```python
from build123d import *

# Parameters (mm, degrees)
BOSS_EXTRUDE1_DEPTH     = 3
BOSS_EXTRUDE1_2_DEPTH   = 3
BOSS_EXTRUDE2_START     = 1.2
SKETCH3_R               = 16.55
SKETCH3_R_2             = 1.65
BOSS_EXTRUDE2_DEPTH     = 1.2
CUT_EXTRUDE1_DEPTH      = 7.2
CUT_EXTRUDE1_DEPTH_BACK = 1.2
SKETCH5_R               = 15.65
CUT_EXTRUDE2_DEPTH      = 7.2


with BuildPart() as part:
    # Sketch2 → Boss-Extrude1 (new body)
    with BuildSketch(Plane.XY):
        with BuildLine():
            ThreePointArc((-3.097702158, 4.826453317), (-4.728295227, 7.32932211), (-5.843255553, 10.100612318))
            Line((-5.843255553, 10.100612318), (-7.089846629, 10.100612318))
            ThreePointArc((-7.089846629, 10.100612318), (-5.792708227, 6.775223774), (-3.812717425, 3.805305689))
            Line((-3.812717425, 3.805305689), (-3.097702158, 4.826453317))
        make_face()
    extrude(amount=BOSS_EXTRUDE1_DEPTH)



with BuildPart() as body_2:
    # Sketch2 → Boss-Extrude1 2 (new body)
    with BuildSketch(Plane.XY):
        with BuildLine():
            Line((-7.089846629, 18.733714328), (-5.843255553, 18.733714328))
            ThreePointArc((-5.843255553, 18.733714328), (11.067705083, 29.611518377), (24.237321062, 14.417163323))
            ThreePointArc((24.237321062, 14.417163323), (17.837317684, 1.946395084), (3.974121001, -0.125290568))
            Line((3.974121001, -0.125290568), (3.259105735, -1.146438196))
            ThreePointArc((3.259105735, -1.146438196), (18.394043324, 0.870033301), (25.437321062, 14.417163323))
            ThreePointArc((25.437321062, 14.417163323), (11.064518196, 30.823330232), (-7.089846629, 18.733714328))
        make_face()
    extrude(amount=BOSS_EXTRUDE1_2_DEPTH)


with BuildPart() as part_1:
    add(part.part)

    add(body_2.part)  # Boss-Extrude2 merges body 2
    # Sketch3 → Boss-Extrude2 (add)
    with BuildSketch(Plane(origin=(0, 0, 0), x_dir=(-1, 0, 0), z_dir=(0, 0, -1)).offset(BOSS_EXTRUDE2_START)):
        with Locations((-8.887321062, 14.417163323)):
            Circle(SKETCH3_R)
        with Locations((-8.887321062, 14.417163323)):
            Circle(SKETCH3_R_2, mode=Mode.SUBTRACT)
    extrude(amount=-BOSS_EXTRUDE2_DEPTH)

    # Sketch4 → Cut-Extrude1 (cut, two sides: drawn at the far end of the back side and taken through both)
    with BuildSketch(Plane.XY.offset(-CUT_EXTRUDE1_DEPTH_BACK)):
        with BuildLine():
            Line((2.037321062, 11.267163323), (2.037321062, 17.567163323))
            Line((2.037321062, 17.567163323), (-6.135994151, 17.567163323))
            ThreePointArc((-6.135994151, 17.567163323), (-6.462678938, 14.417163323), (-6.135994151, 11.267163323))
            Line((-6.135994151, 11.267163323), (2.037321062, 11.267163323))
        make_face()
        with BuildLine():
            ThreePointArc((-6.135994151, 11.267163323), (-6.462678938, 14.417163323), (-6.135994151, 17.567163323))
            Line((-6.135994151, 17.567163323), (-7.360140278, 17.567163323))
            ThreePointArc((-7.360140278, 17.567163323), (-7.662678938, 14.417163323), (-7.360140278, 11.267163323))
            Line((-7.360140278, 11.267163323), (-6.135994151, 11.267163323))
        make_face()
        with BuildLine():
            Line((2.148489026, -0.698743623), (2.850630399, 0.304018179))
            ThreePointArc((2.850630399, 0.304018179), (0.082922764, 1.843179443), (-2.31002748, 3.917549728))
            Line((-2.31002748, 3.917549728), (-3.012168853, 2.914787926))
            ThreePointArc((-3.012168853, 2.914787926), (-0.605368959, 0.86019699), (2.148489026, -0.698743623))
        make_face()
        with BuildLine():
            Line((7.538651413, 6.999206045), (2.377993534, 10.612737594))
            Line((2.377993534, 10.612737594), (-2.31002748, 3.917549728))
            ThreePointArc((-2.31002748, 3.917549728), (0.082922764, 1.843179443), (2.850630399, 0.304018179))
            Line((2.850630399, 0.304018179), (7.538651413, 6.999206045))
        make_face()
        with BuildLine():
            Line((2.377993534, 10.612737594), (2.037321062, 11.267163323))
            Line((2.037321062, 11.267163323), (-6.135994151, 11.267163323))
            ThreePointArc((-6.135994151, 11.267163323), (-4.728295227, 7.32932211), (-2.31002748, 3.917549728))
            Line((-2.31002748, 3.917549728), (2.377993534, 10.612737594))
        make_face()
        with BuildLine():
            ThreePointArc((-2.31002748, 3.917549728), (-4.728295227, 7.32932211), (-6.135994151, 11.267163323))
            Line((-6.135994151, 11.267163323), (-7.360140278, 11.267163323))
            ThreePointArc((-7.360140278, 11.267163323), (-5.792708227, 6.775223774), (-3.012168853, 2.914787926))
            Line((-3.012168853, 2.914787926), (-2.31002748, 3.917549728))
        make_face()
    extrude(amount=CUT_EXTRUDE1_DEPTH + CUT_EXTRUDE1_DEPTH_BACK, mode=Mode.SUBTRACT)

    # Sketch5 → Cut-Extrude2 (cut)
    with BuildSketch(Plane.XY):
        with Locations((8.887321062, 14.417163323)):
            Circle(SKETCH5_R)
    extrude(amount=CUT_EXTRUDE2_DEPTH, mode=Mode.SUBTRACT)


solid = part_1.part
```
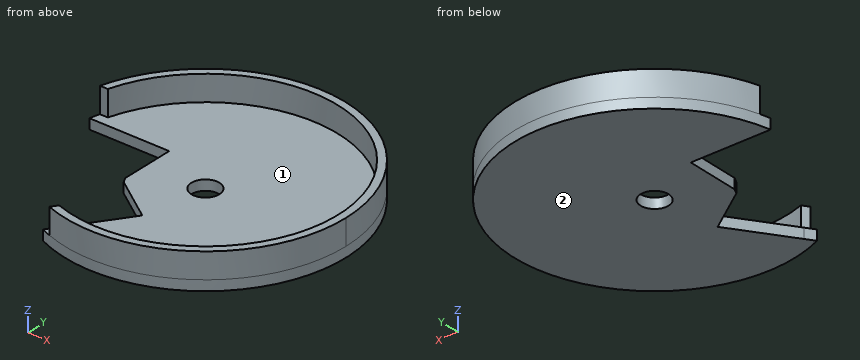
Verification items for the finished model (mm, model axes). Face numbers are marked on the shaded views. Coordinates: 2 decimals unless noted, no trailing zeros. Loops run counter-clockwise (first coordinate to the right, second up) from the corner with the lowest first, then second, coordinate; pieces in that order, holes last. Notation, with made-up numbers: (1.5, 59.5) -> (41.5, 59.5) arc R21 ccw to (41.5, 83.5) -> close; hole circle Ø11 at (34.5, 23). An arc over 180 degrees is marked (long way). Answer in a Markdown table with one row per item.
1) Draft check along X on the marked faces 1 and 2. Enter one of: released by +X, released by -X, zero draft, split by the parting line, or undercut.
The answers:
| item | result |
|---|---|
| face 1 | undercut |
| face 2 | zero draft |
2) Depth check by flat-ended pin: P1, Ø5.5, axis at x = 8.89, y = 14.42, coming from the +Z side; P2, Ø0.5, axis at x = -6.5, z = 2, coming from the -Y side; P3, Ø2, axis at x = 1, y = 15.5, coming from the +Z side; P4, Ø19, axis at x = 8.89, y = 14.42, coming from the -Z side. Enter the tip coordinate at first touch or a pass-through.
The answers:
| item | result |
|---|---|
| P1 | stops at z = 0 |
| P2 | stops at y = 18.73 |
| P3 | passes through |
| P4 | stops at z = -1.2 |
3) Section check D-D (z = 2.5). Record the cut outline in (x, y).
The answers:
| item | result |
|---|---|
| outline | (-7.09, 18.73) -> (-6.16, 18.73) arc R15.65 cw (long way) to (3.79, -0.38) -> (3.26, -1.15) arc R16.55 ccw (long way) to start |
4) Section check A-A (z = -0.75). Record the cut outline in (x, y), and give its area (3 significant figures).
The answers:
| item | result |
|---|---|
| outline | (-7.36, 17.57) -> (2.04, 17.57) -> (2.04, 11.27) -> (2.38, 10.61) -> (7.54, 7) -> (2.15, -0.7) arc R16.55 ccw (long way) to start; hole circle Ø3.3 at (8.89, 14.42) |
| area | 684 mm2 |
5) Section check C-C (y = 20). Record the cut outline in (x, z), and give its area (3 significant figures).
The answers:
| item | result |
|---|---|
| outline | (-6.69, -1.2) -> (24.47, -1.2) -> (24.47, 3) -> (23.51, 3) -> (23.51, 0) -> (-5.73, 0) -> (-5.73, 3) -> (-6.69, 3) -> close |
| area | 43.1 mm2 |
6) Section check B-B (x = 6.5). Record the cut outline in (y, z), and give its area (3 significant figures).
The answers:
| item | result |
|---|---|
| outline | (-1.96, -1.2) -> (5.52, -1.2) -> (5.52, 0) -> (-1.05, 0) -> (-1.05, 3) -> (-1.96, 3) -> close; (7.73, -1.2) -> (30.79, -1.2) -> (30.79, 3) -> (29.88, 3) -> (29.88, 0) -> (7.73, 0) -> close |
| area | 42.1 mm2 |
7) Scan lines: line 1 along Y through (x, z) = (8.5, 1.95); line 2 along Z through (x, y) = (21, 8); line 3 along Y through (x, z) = (6.5, 0.05). Record each from-to range of solid material in increasing order. Write a range as from..to.
The answers:
| item | result |
|---|---|
| line 1 | y = -2.13..-1.23, 30.06..30.96 |
| line 2 | z = -1.2..0 |
| line 3 | y = -1.96..-1.05, 29.88..30.79 |
